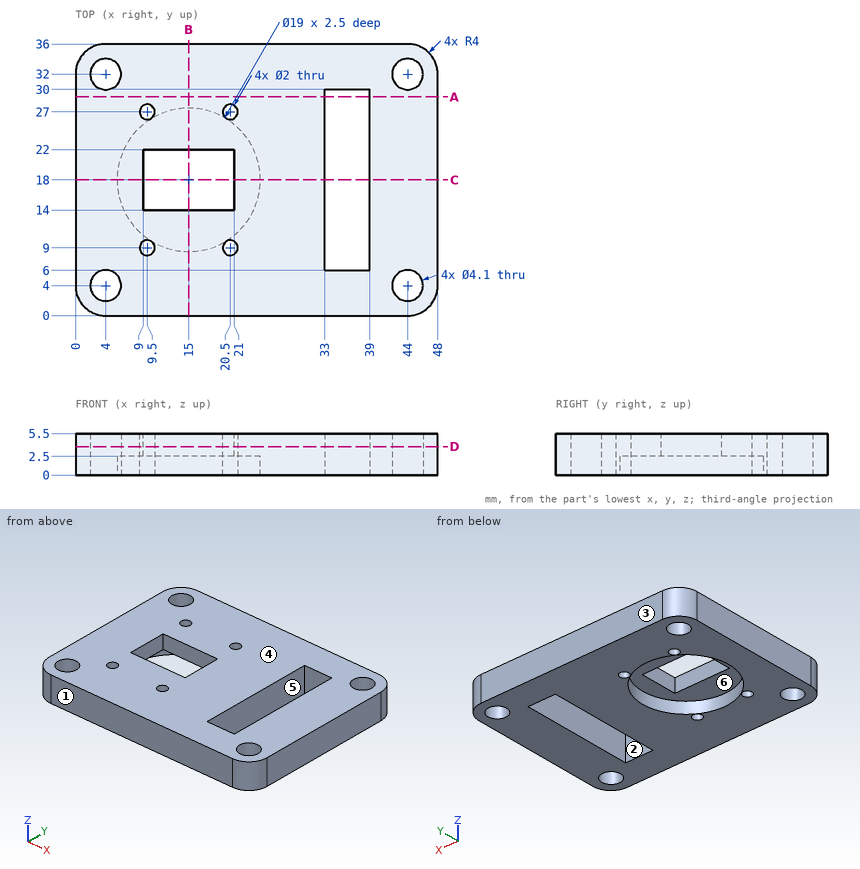
For this review, use the dimensioned drawing (mm, ordinates from the lowest corner) and the shaded views. A direction names the side the tool comes from. Round coordinates to 2 decimals unless told otherwise and drop trailing zeros. Write each loop counter-clockwise with the first axis right and the second up, starting at its lowest first coordinate (ties: lowest second). Pieces come first, ordered by that corner, then holes. Notation, with made-up numbers: (9.5, 21.25) -> (21.5, 21.25) arc R18 ccw to (21.5, 54.25) -> close; hole circle Ø11 at (-39, 29). An arc over 180 degrees is marked (long way). Use one line per item in the form item = value.
Q1. To check wall thickness, follow probe 1 along Y at (x, z) = (9.5, 3.45); probe 2 along Y at (x, z) = (4, 3.65); probe 3 along Y at (x, z) = (37.5, 4.4). State the ranges of each line that lie inside material, in increasing order. Write a range as from..to.
Resolved:
probe_1 = 0..8, 10..14, 22..26, 28..36
probe_2 = 0..1.95, 6.05..29.95, 34.05..36
probe_3 = 0..6, 30..36
Q2. The part is to be moulded in two halves that separate along Y. For the marked faces 1, 2 and 3, say which applies: released by +Y, released by -Y, zero draft, split by the parting line, or undercut.
Resolved:
face_1 = released by -Y
face_2 = undercut
face_3 = released by +Y
Q3. Clearance check with a flat-ended pin moving along its axis: pin 1 Ø1.6 at (x, y) = (9.5, 27) entering from +Z. State where the tip first meets the part, or that it passes through.
Resolved:
pin_1 = through
Q4. Consider section B-B (x = 15). State the section outline as (y, z) points.
Resolved:
outline = (0, 0) -> (8.5, 0) -> (8.5, 2.5) -> (14, 2.5) -> (14, 5.5) -> (0, 5.5) -> close; (22, 2.5) -> (27.5, 2.5) -> (27.5, 0) -> (36, 0) -> (36, 5.5) -> (22, 5.5) -> close
Q5. Consider section D-D (z = 3.8). State how many separate pieces and enclosed holes the cut face has, then the cut area to 3 significant figures.
Resolved:
separate_pieces = 1
enclosed_holes = 10
area = 1,410 mm²
Q6. Machinability: for the marked faces 4, 5 and 6, which of the approach directions +Z, -Z, +X, -X, +Y, -Y give a long, thin tool a straight path to every point of the face, cutting with its end or side? Answer none if there is none.
Resolved:
face_4 = +Z, +X, -X, +Y, -Y
face_5 = +Z, -Z
face_6 = -Z
Q7. Consider section A-A (y = 29). State the section outline as (x, z) points, then the cut area to 3 significant figures.
Resolved:
outline = (0, 0) -> (33, 0) -> (33, 5.5) -> (0, 5.5) -> close; (39, 0) -> (48, 0) -> (48, 5.5) -> (39, 5.5) -> close
area = 231 mm²
Q8. Consider section C-C (y = 18). State the section outline as (x, z) points, then the cut area to 4 significant figures.
Resolved:
outline = (0, 0) -> (5.5, 0) -> (5.5, 2.5) -> (9, 2.5) -> (9, 5.5) -> (0, 5.5) -> close; (21, 2.5) -> (24.5, 2.5) -> (24.5, 0) -> (33, 0) -> (33, 5.5) -> (21, 5.5) -> close; (39, 0) -> (48, 0) -> (48, 5.5) -> (39, 5.5) -> close
area = 147.5 mm²
